from build123d import *

# Parameters (mm, degrees)
SKETCH1_R            = 60
SKETCH1_R_2          = 23.5
BOSS_EXTRUDE1_DEPTH  = 5
M6_CLEARANCE_HOLE1_D = 6.6


with BuildPart() as part:
    # Sketch1 → Boss-Extrude1 (new body)
    with BuildSketch(Plane(origin=(0, 0, 0), x_dir=(1, 0, 0), z_dir=(0, 1, 0))):
        Circle(SKETCH1_R)
        Circle(SKETCH1_R_2, mode=Mode.SUBTRACT)
    extrude(amount=BOSS_EXTRUDE1_DEPTH)

    # M6 Clearance Hole1 (through all)
    with Locations(Plane(origin=(0, 5, 0), x_dir=(1, 0, 0), z_dir=(0, 1, 0))):
        with Locations((-37.476659403, 37.476659403), (0, 53), (37.476659403, 37.476659403), (53, 0), (37.476659403, -37.476659403), (0, -53), (-37.476659403, -37.476659403), (-53, 0)):
            Hole(M6_CLEARANCE_HOLE1_D / 2)


solid = part.part
Input: part model. Units: mm. Frame: model coordinates. Give positions to 0.01 mm unless a question says otherwise; leave off trailing zeros. Order: outer loops, then holes, each group sorted by start corner. A loop starts at its lowest first (then second) coordinate and runs counter-clockwise, first axis right, second up.
Q1. Draft query along X for faces 1 (the flat face through (26, 0, -1)), 2 (the cylindrical face through (35.95, 2.47, -34.55)), 3 (the cylindrical face through (-40.525, 2.465, 38.741)), 4 (the cylindrical face through (-59.94, 2.46, -2.64)). Return one class per face: +X half, -X half, draft (parallel to the pull), parting line (faces both ways), or undercut.
Checked values:
face 1: draft
face 2: undercut
face 3: undercut
face 4: parting line
Q2. Contact query for flat-ended pins moving along their axis: pin 1 Ø5.5 at (x, z) = (37.48, -37.48) entering from +Y; pin 2 Ø1 at (y, z) = (4.5, -19) entering from -X; pin 3 Ø1 at (y, z) = (1.5, -44) entering from -X. Output: stop coordinate, or through.
Checked values:
pin 1: passes through
pin 2: stops at x = -57.08
pin 3: stops at x = -41.32
Q3. Ray query, probe 1 along Z at (x, y) = (0, 2.2); probe 2 along X at (y, z) = (4.3, 2.5); probe 3 along X at (y, z) = (4.7, -39). Return the intervals inside material, ascending.
Checked values:
probe 1: z = -60 to -56.3, -49.7 to -23.5, 23.5 to 49.7, 56.3 to 60
probe 2: x = -59.95 to -55.15, -50.85 to -23.37, 23.37 to 50.85, 55.15 to 59.95
probe 3: x = -45.6 to -40.4, -34.55 to 34.55, 40.4 to 45.6
Q4. Section B-B on z = 0. Output: boundary loops of the cut face in (x, y), and give its area (3 significant figures).
Checked values:
outline: (-60, 0) - (-56.3, 0) - (-56.3, 5) - (-60, 5) - close; (-49.7, 0) - (-23.5, 0) - (-23.5, 5) - (-49.7, 5) - close; (23.5, 0) - (49.7, 0) - (49.7, 5) - (23.5, 5) - close; (56.3, 0) - (60, 0) - (60, 5) - (56.3, 5) - close
area: 299 mm2
Q5. Section A-A on x = 0. Output: boundary loops of the cut face in (y, z).
Checked values:
outline: (0, -60) - (5, -60) - (5, -56.3) - (0, -56.3) - close; (0, -49.7) - (5, -49.7) - (5, -23.5) - (0, -23.5) - close; (0, 23.5) - (5, 23.5) - (5, 49.7) - (0, 49.7) - close; (0, 56.3) - (5, 56.3) - (5, 60) - (0, 60) - close
Q6. Section D-D on x = -12. Output: boundary loops of the cut face in (y, z), and give its area (3 significant figures).
Checked values:
outline: (0, -58.79) - (5, -58.79) - (5, -20.21) - (0, -20.21) - close; (0, 20.21) - (5, 20.21) - (5, 58.79) - (0, 58.79) - close
area: 386 mm2
Q7. Section C-C on z = 17.5. Output: boundary loops of the cut face in (x, y).
Checked values:
outline: (-57.39, 0) - (-15.68, 0) - (-15.68, 5) - (-57.39, 5) - close; (15.68, 0) - (57.39, 0) - (57.39, 5) - (15.68, 5) - close
